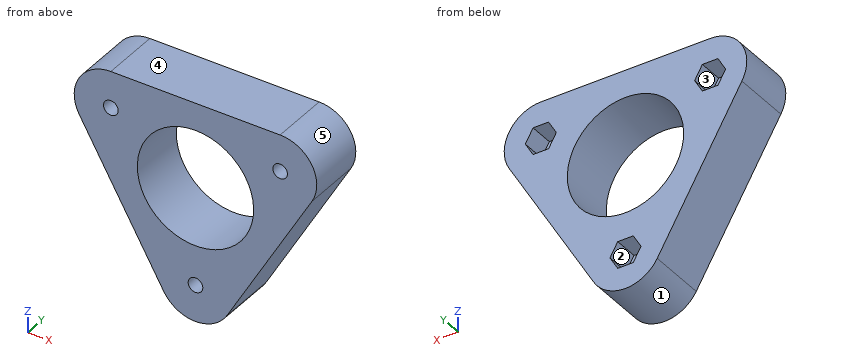
```python
from build123d import *

# Parameters (mm, degrees)
ESQUISSE1_R             = 11.9
ESQUISSE1_R_2           = 1.5
BOSS_EXTRU_1_DEPTH      = 12
ENL_V_MAT_EXTRU_1_DEPTH = 5


with BuildPart() as part:
    # Esquisse1 → Boss.-Extru.1 (new body)
    with BuildSketch(Plane(origin=(0, 0, 0), x_dir=(1, 0, 0), z_dir=(0, 1, 0))):
        with BuildLine():
            Line((-6.495190528, 23.75), (-23.815698604, -6.25))
            ThreePointArc((-23.815698604, -6.25), (-23.815698604, -13.75), (-17.320508076, -17.5))
            Line((-17.320508076, -17.5), (17.320508076, -17.5))
            ThreePointArc((17.320508076, -17.5), (23.815698604, -13.75), (23.815698604, -6.25))
            Line((23.815698604, -6.25), (6.495190528, 23.75))
            ThreePointArc((6.495190528, 23.75), (0, 27.5), (-6.495190528, 23.75))
        make_face()
        with Locations(Location((0, 0, 0), (0, 0, 270))):
            Circle(ESQUISSE1_R, mode=Mode.SUBTRACT)
        with Locations(Location((-17.320508076, -10, 0), (0, 0, 270))):
            Circle(ESQUISSE1_R_2, mode=Mode.SUBTRACT)
        with Locations(Location((0, 20, 0), (0, 0, 270))):
            Circle(ESQUISSE1_R_2, mode=Mode.SUBTRACT)
        with Locations(Location((17.320508076, -10, 0), (0, 0, 270))):
            Circle(ESQUISSE1_R_2, mode=Mode.SUBTRACT)
    extrude(amount=BOSS_EXTRU_1_DEPTH)

    # Esquisse2 → Enlèv. mat.-Extru.1 (cut)
    with BuildSketch(Plane(origin=(0, 12, 0), x_dir=(1, 0, 0), z_dir=(0, 1, 0))):
        Polygon((-18.908221316, -7.25), (-20.495934556, -10), (-18.908221316, -12.75), (-15.732794835, -12.75), (-14.145081595, -10), (-15.732794835, -7.25), align=None)
        Polygon((-1.58771324, 22.75), (-3.175426481, 20), (-1.58771324, 17.25), (1.58771324, 17.25), (3.175426481, 20), (1.58771324, 22.75), align=None)
        Polygon((18.908221316, -7.25), (15.732794835, -7.25), (14.145081595, -10), (15.732794835, -12.75), (18.908221316, -12.75), (20.495934556, -10), align=None)
    extrude(amount=-ENL_V_MAT_EXTRU_1_DEPTH, mode=Mode.SUBTRACT)


solid = part.part
```
Verification items for the finished model (mm, model axes). Face numbers are marked on the shaded views. A direction names the side the tool comes from. Give positions to 0.01 mm unless a question says otherwise; leave off trailing zeros. Order: outer loops, then holes, each group sorted by start corner. A loop starts at its lowest first (then second) coordinate and runs counter-clockwise, first axis right, second up. Notation, with made-up numbers: (41, -13.75) -> (50, -13.75) arc R20 ccw to (50, 12.25) -> close; hole circle Ø5 at (39, 71). An arc over 180 degrees is marked (long way). One line per item, written item: value.
(1) Sectioned sample at A-A on y = 4.75. Record the cut outline in (x, z), then the cut area to 3 significant figures.
Final values:
outline: (-23.82, 6.25) -> (-6.5, -23.75) arc R7.5 ccw to (6.5, -23.75) -> (23.82, 6.25) arc R7.5 ccw to (17.32, 17.5) -> (-17.32, 17.5) arc R7.5 ccw to start; hole circle Ø3 at (-17.32, 10); hole circle Ø23.8 at (0, 0); hole circle Ø3 at (0, -20); hole circle Ø3 at (17.32, 10)
area: 1,010 mm^2
(2) Sectioned sample at D-D on x = 5.5. Record the cut outline in (y, z).
Final values:
outline: (0, -25.1) -> (12, -25.1) -> (12, -10.55) -> (0, -10.55) -> close; (0, 10.55) -> (12, 10.55) -> (12, 17.5) -> (0, 17.5) -> close
(3) Sectioned sample at B-B on x = 0. Record the cut outline in (y, z).
Final values:
outline: (0, -27.5) -> (12, -27.5) -> (12, -22.75) -> (7, -22.75) -> (7, -21.5) -> (0, -21.5) -> close; (0, -18.5) -> (7, -18.5) -> (7, -17.25) -> (12, -17.25) -> (12, -11.9) -> (0, -11.9) -> close; (0, 11.9) -> (12, 11.9) -> (12, 17.5) -> (0, 17.5) -> close
(4) Scan lines: line 1 along X through (y, z) = (5.5, 10); line 2 along X through (y, z) = (9.5, 11); line 3 along Z through (x, y) = (-1, 1.25). Record each from-to range of solid material in increasing order. Write a range as [from, to].
Final values:
line 1: [-24.82, -18.82], [-15.82, -6.45], [6.45, 15.82], [18.82, 24.82]
line 2: [-24.75, -19.92], [-14.72, -4.54], [4.54, 14.72], [19.92, 24.75]
line 3: [-27.43, -21.12], [-18.88, -11.86], [11.86, 17.5]
(5) Tool access check on the marked faces 1 and 2. Record the directions out of +Z, -Z, +X, -X, +Y, -Y that give a thin tool (end or side, any length) a straight path to the whole face; none if there is none.
Final values:
face 1: -Z, +Y, -Y
face 2: +Y
(6) Sectioned sample at C-C on z = 0. Record the cut outline in (x, y).
Final values:
outline: (-20.21, 0) -> (-11.9, 0) -> (-11.9, 12) -> (-20.21, 12) -> close; (11.9, 0) -> (20.21, 0) -> (20.21, 12) -> (11.9, 12) -> close
(7) Gauge pin test, flat ends, axial feed: pin 1 (2 mm diameter, centred on x = -2.5, y = 5.5, fed in from -Z); pin 2 (3.5 mm diameter, centred on x = 17, y = 10.5, fed in from -Z); pin 3 (1 mm diameter, centred on y = 5.5, z = -21, fed in from -X). Record the tip position at first contact, or that the pin passes through.
Final values:
pin 1: z = -27.35
pin 2: z = -8.59
pin 3: x = -8.37
(8) Draft check along Z on the marked faces 3, 4 and 5. Enter one of: pulls with the +Z half, pulls with the -Z half, needs draft (parallel to the pull), parting line crosses it, or undercut.
Final values:
face 3: undercut
face 4: pulls with the +Z half
face 5: parting line crosses it
